Geometry check sheet. Reference: the model listing, model coordinates, mm. Face numbers are marked on the shaded views. A direction names the side the tool comes from. Give positions to 0.01 mm unless a question says otherwise; leave off trailing zeros. Order: outer loops, then holes, each group sorted by start corner. A loop starts at its lowest first (then second) coordinate and runs counter-clockwise, first axis right, second up. Notation, with made-up numbers: M 34,81 L 76,81 A20 ccw 76,103 Z; hole C -3,12.25 d11. An arc over 180 degrees is marked long. One line per question, with ' | ' between items. Start each with the question number.
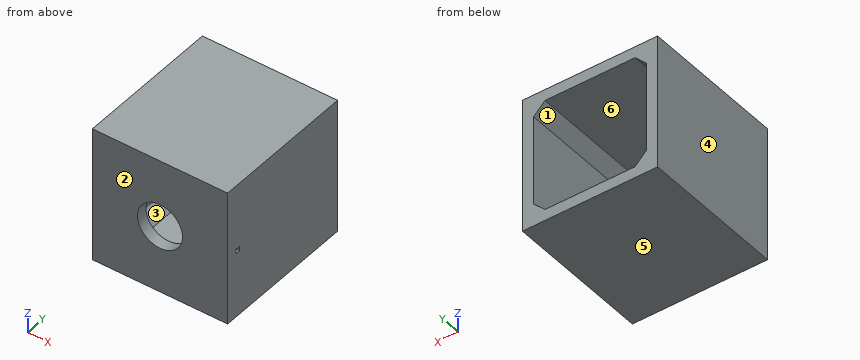
from build123d import *

# Parameters (mm, degrees)
SKETCH1_W           = 60
SKETCH1_H           = 60
SKETCH1_W_2         = 50
SKETCH1_H_2         = 50
BOSS_EXTRUDE1_DEPTH = 60
SKETCH2_W           = 60
SKETCH2_H           = 60
BOSS_EXTRUDE2_DEPTH = 5
SKETCH3_R           = 10
CUT_EXTRUDE1_DEPTH  = 6
CHAMFER4_SIZE       = 5
SKETCH7_W           = 2
SKETCH7_H           = 2
CUT_EXTRUDE3_DEPTH  = 5


with BuildPart() as part:
    # Sketch1 → Boss-Extrude1 (new body)
    with BuildSketch(Plane(origin=(0, 0, 0), x_dir=(1, 0, 0), z_dir=(0, 1, 0))):
        Rectangle(SKETCH1_W, SKETCH1_H)
        Rectangle(SKETCH1_W_2, SKETCH1_H_2, mode=Mode.SUBTRACT)
    extrude(amount=BOSS_EXTRUDE1_DEPTH)

    # Sketch2 → Boss-Extrude2 (add)
    with BuildSketch(Plane.XZ):
        Rectangle(SKETCH2_W, SKETCH2_H)
    extrude(amount=BOSS_EXTRUDE2_DEPTH)

    # Sketch3 → Cut-Extrude1 (cut, through all)
    with BuildSketch(Plane(origin=(0, 0, 0), x_dir=(1, 0, 0), z_dir=(0, 1, 0))):
        Circle(SKETCH3_R)
    extrude(amount=-CUT_EXTRUDE1_DEPTH, mode=Mode.SUBTRACT)

    # Chamfer4
    chamfer4_edges = [part.edges().sort_by_distance(p)[0] for p in [
        (25, 30, 25),
        (25, 30, -25),
        (-25, 30, -25),
        (-25, 30, 25),
    ]]
    chamfer(chamfer4_edges, length=CHAMFER4_SIZE)

    # Sketch7 → Cut-Extrude3 (cut)
    with BuildSketch(Plane.ZY.offset(-25)):
        with Locations((0, 1)):
            Rectangle(SKETCH7_W, SKETCH7_H)
    extrude(amount=-CUT_EXTRUDE3_DEPTH, mode=Mode.SUBTRACT)


solid = part.part
Item 1: Material ranges on line 1 along X through (y, z) = (-1.7, 0); line 2 along X through (y, z) = (31, -6), recorded low to high.
Item 2: Cross-section at B-B, the plane x = 0. Record the cut outline in (y, z).
Item 3: Cross-section at A-A, the plane z = 0. Record the cut outline in (x, y), plus the area to 3 significant figures.
Item 4: Cross-section at C-C, the plane y = 17. Record the cut outline in (x, z).
Item 5: Cross-section at D-D, the plane x = -17. Record the cut outline in (y, z), plus the area to 3 significant figures.
Item 6: Mould release check, pull along X, two halves, no side actions. Record for the marked faces 3, 4, 5 and 6: released by +X, released by -X, zero draft, split by the parting line, or undercut.
Item 7: Set-up check for the marked faces 1 and 2: record each of +Z, -Z, +X, -X, +Y, -Y from which the full face is reachable in a straight line by a thin tool's end or side.
Item 8: Depth check by flat-ended pin: pin 1 (4 mm diameter, centred on x = 1, z = 11.5, fed in from +Y). Enter the tip coordinate at first touch or a pass-through.
Outcome:
1) line 1: x = -30 to -10, 10 to 30 | line 2: x = -30 to -25, 25 to 30
2) outline: M -5,-30 L 60,-30 L 60,-25 L 0,-25 L 0,-10 L -5,-10 Z; M -5,10 L 0,10 L 0,25 L 60,25 L 60,30 L -5,30 Z
3) outline: M -30,-5 L -10,-5 L -10,0 L -25,0 L -25,60 L -30,60 Z; M 10,-5 L 30,-5 L 30,0 L 10,0 Z; M 25,2 L 30,2 L 30,60 L 25,60 Z | area: 790 mm²
4) outline: M -30,-30 L 30,-30 L 30,30 L -30,30 Z; hole M -25,-20 L -20,-25 L 20,-25 L 25,-20 L 25,20 L 20,25 L -20,25 L -25,20 Z
5) outline: M -5,-30 L 60,-30 L 60,-25 L 0,-25 L 0,25 L 60,25 L 60,30 L -5,30 Z | area: 900 mm²
6) face 3: undercut | face 4: released by -X | face 5: zero draft | face 6: undercut
7) face 1: +Y | face 2: +Z, -Z, +X, -X, -Y
8) pin 1: stops at y = 0
